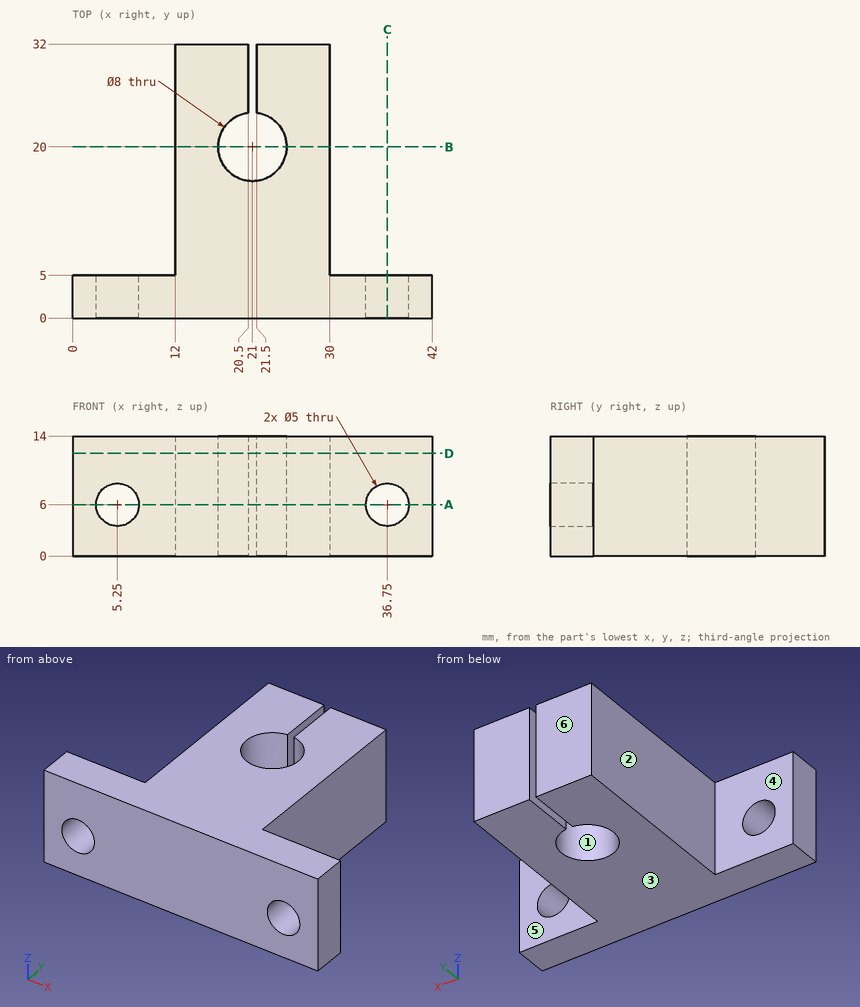
Geometry check sheet. Reference: drawing and pictorial views, mm from the part's lowest x, y, z. A direction names the side the tool comes from. Give positions to 0.01 mm unless a question says otherwise; leave off trailing zeros. Order: outer loops, then holes, each group sorted by start corner. A loop starts at its lowest first (then second) coordinate and runs counter-clockwise, first axis right, second up. Notation, with made-up numbers: (81.25, 55.5) -> (97.25, 55.5) arc R26 cw to (97.25, 73.5) -> close; hole circle Ø5 at (-36, 87.25). An arc over 180 degrees is marked (long way). Write each question's results on one line, items separated by ' | '. Start each with the question number.
(1) Access from +Z, -Z, +X, -X, +Y, -Y to the whole of each face (thin tool, end or side, straight path). Record for the marked faces 4, 5 and 6.
(2) Sectioned sample at C-C (x = 36.75). Enter the section's corners in (y, z).
(3) Sectioned sample at D-D (z = 12). Enter the section's corners in (x, y).
(4) Gauge pin test, flat ends, axial feed: P1, Ø7, axis at y = 22.5, z = 9.5, coming from the +X side; P2, Ø8, axis at x = 5.25, z = 6, coming from the +Y side; P3, Ø1, axis at y = 23, z = 10, coming from the -X side. Record the tip position at first contact, or that the pin passes through.
(5) Mould release check, pull along X, two halves, no side actions. Record for the marked faces 1, 2 and 3: pulls with the +X half, pulls with the -X half, needs draft (parallel to the pull), parting line crosses it, or undercut.
(6) Sectioned sample at A-A (z = 6). Enter the section's corners in (x, y).
(7) Sectioned sample at B-B (y = 20). Enter the section's corners in (x, z).
(8) Scan lines: line 1 (X direction, y = 2.5, z = 6); line 2 (X direction, y = 28.5, z = 13.5); line 3 (X direction, y = 10.5, z = 12). Record each from-to range of solid material in increasing order.
Answer below:
1) face 4: +Z, -Z, -X, +Y | face 5: +Z, -Z, +X, +Y | face 6: +Z, -Z, +X, -X, +Y
2) outline: (0, 0) -> (5, 0) -> (5, 3.5) -> (0, 3.5) -> close; (0, 8.5) -> (5, 8.5) -> (5, 14) -> (0, 14) -> close
3) outline: (0, 0) -> (42, 0) -> (42, 5) -> (30, 5) -> (30, 32) -> (21.5, 32) -> (21.5, 23.97) arc R4 cw (long way) to (20.5, 23.97) -> (20.5, 32) -> (12, 32) -> (12, 5) -> (0, 5) -> close
4) P1: x = 30 | P2: y = 5 | P3: x = 12
5) face 1: undercut | face 2: pulls with the -X half | face 3: needs draft
6) outline: (0, 0) -> (2.75, 0) -> (2.75, 5) -> (0, 5) -> close; (7.75, 0) -> (34.25, 0) -> (34.25, 5) -> (30, 5) -> (30, 32) -> (21.5, 32) -> (21.5, 23.97) arc R4 cw (long way) to (20.5, 23.97) -> (20.5, 32) -> (12, 32) -> (12, 5) -> (7.75, 5) -> close; (39.25, 0) -> (42, 0) -> (42, 5) -> (39.25, 5) -> close
7) outline: (12, 0) -> (17, 0) -> (17, 14) -> (12, 14) -> close; (25, 0) -> (30, 0) -> (30, 14) -> (25, 14) -> close
8) line 1: 0 to 2.75, 7.75 to 34.25, 39.25 to 42 | line 2: 12 to 20.5, 21.5 to 30 | line 3: 12 to 30
